Here's how the part is built. I have some questions about the finished solid (model axes, mm). Face numbers are marked on the shaded views. A direction names the side the tool comes from. Give positions to 0.01 mm unless a question says otherwise; leave off trailing zeros. Loops run counter-clockwise (first coordinate to the right, second up) from the corner with the lowest first, then second, coordinate; pieces in that order, holes last. Notation, with made-up numbers: M 0,45.25 L 44,45.25 A29 cw 44,65.25 Z; hole C 82.5,62.25 d10. An arc over 180 degrees is marked long. Answer as CSV lines item,"result". Start each with the question number.
Item 1: I want a section at C-C on z = -36.5. List the corners of the cut face in (x, y) for me (3 decimals).
Item 2: If I drill on line 1 along Y through (x, z) = (-24.25, -28) (3 decimals); line 2 along Z through (x, y) = (-21, -20); line 3 along X through (y, z) = (-4, -35), over which ranges is the centre line in solid material (lowest first)? Write a range as from..to.
Item 3: I want a section at B-B on z = -30.25. List the corners of the cut face in (x, y) for me (3 decimals), plus the area to 3 significant figures.
Item 4: For the marked faces 1, 2, 3 and 4, which set-ups out of +Z, -Z, +X, -X, +Y, -Y let a thin tool reach every point of the face, with its end or its side?
Item 5: I want a section at D-D on y = -18.75. List the corners of the cut face in (x, z) for me, plus the area to 3 significant figures.
Item 6: I want a section at A-A on y = -14.25. List the corners of the cut face in (x, z) for me.
Item 7: Will these pins go through, and if not, where does the flat tip stop? P1, Ø4, axis at x = -27, y = -10, coming from the +Z side; P2, Ø1.5, axis at y = -9, z = -29, coming from the -X side.
Item 8: If we mould it in two halves opening along Y, with no side actions, what happens to the marked faces 5, 6, 7 and 8? For each: released by +Y, released by -Y, zero draft, split by the parting line, or undercut.
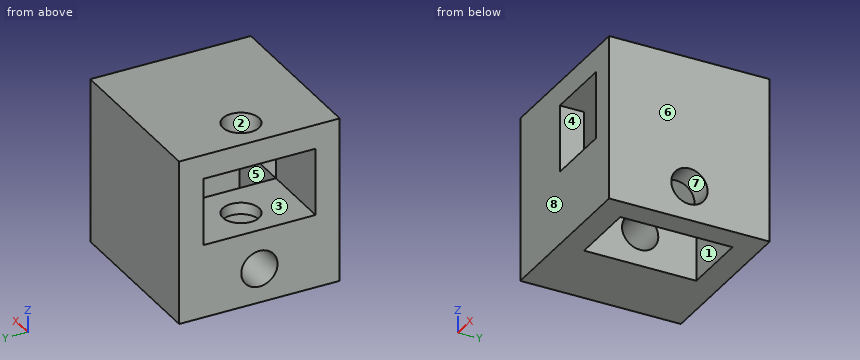
from build123d import *

# Parameters (mm, degrees)
F0_W     = 21.6662
F0_H     = 21.6662
F1_DEPTH = 3.175
F2_W     = 18.4912
F2_H     = 3.175
F2_W_2   = 9.652
F2_H_2   = 9.652
F3_DEPTH = 14.732
F5_DEPTH = 13.5382
F7_DEPTH = 25.4
F9_DEPTH = 3.175


# Not quite as in the source:
# - a length typed as a fraction of an inch, garbled in the dataset ("3 / 203.2 mm" for 3/8 in), is restored


with BuildPart() as f1:
    # F0 (on Front) → F1 (new body)
    with BuildSketch(Plane.XZ):
        with Locations((-21.4400560975, -33.0820980474)):
            Rectangle(F0_W, F0_H)
    extrude(amount=F1_DEPTH)

    # F2 (on face) → F3 (join)
    with BuildSketch(Plane.XZ.offset(3.175)):
        with Locations((-23.0275560975, -23.8364980474)):
            Rectangle(F2_W, F2_H)
        Polygon((-13.7819560975, -22.2489980474), (-13.7819560975, -25.4239980474), (-13.7819560975, -43.9151980474), (-10.6069560975, -43.9151980474), (-10.6069560975, -22.2489980474), align=None)
        with Locations((-27.4471560975, -39.0891980474)):
            Rectangle(F2_W_2, F2_H_2)
    extrude(amount=F3_DEPTH)

    # F4 (on face) → F5 (cut)
    with BuildSketch(Plane.XY.offset(-22.2489980474)):
        with BuildLine():
            ThreePointArc((-25.3961060975, -10.541), (-27.7773560975, -8.15975), (-30.1586060975, -10.541))
            ThreePointArc((-30.1586060975, -10.541), (-27.7773560975, -12.92225), (-25.3961060975, -10.541))
        make_face()
    extrude(amount=-F5_DEPTH, mode=Mode.SUBTRACT)

    # F6 (on face) → F7 (cut)
    with BuildSketch(Plane.YZ.offset(-10.6069560975)):
        with BuildLine():
            ThreePointArc((-8.15975, -39.4193980474), (-12.2247980227, -37.7356000247), (-10.541, -41.8006480474))
            ThreePointArc((-10.541, -41.8006480474), (-8.8572019773, -41.1031960701), (-8.15975, -39.4193980474))
        make_face()
    extrude(amount=-F7_DEPTH, mode=Mode.SUBTRACT)

    # F8 (on face) → F9 (join)
    with BuildSketch(Plane.XZ.offset(17.907)):
        Polygon((-10.6069560975, -43.9151980474), (-10.6069560975, -22.2489980474), (-32.2731560975, -22.2489980474), (-32.2731560975, -25.4239980474), (-22.6211560975, -25.4239980474), (-13.7819560975, -25.4239980474), (-13.7819560975, -34.2631980474), (-13.7819560975, -43.9151980474), align=None)
        Polygon((-22.6211560975, -25.4239980474), (-32.2731560975, -25.4239980474), (-32.2731560975, -43.9151980474), (-13.7819560975, -43.9151980474), (-13.7819560975, -34.2631980474), (-22.6211560975, -34.2631980474), align=None)
    extrude(amount=F9_DEPTH)


solid = f1.part
Result:
1,outline,"M -32.273,-21.082 L -10.607,-21.082 L -10.607,0 L -32.273,0 Z; hole M -22.621,-17.907 L -13.782,-17.907 L -13.782,-3.175 L -22.621,-3.175 Z"
2,line 1,"-21.082..-17.907, -3.175..0"
2,line 2,"-43.92..-34.26, -25.42..-22.25"
2,line 3,"-32.27..-22.62, -13.78..-10.61"
3,outline,"M -32.273,-21.082 L -22.621,-21.082 L -22.621,-17.907 L -32.273,-17.907 Z; M -32.273,-3.175 L -13.782,-3.175 L -13.782,-21.082 L -10.607,-21.082 L -10.607,0 L -32.273,0 Z"
3,area,"156 mm^2"
4,face 1,"none"
4,face 2,"+Z"
4,face 3,"-X"
4,face 4,"-Y"
5,outline,"M -32.27,-43.92 L -10.61,-43.92 L -10.61,-22.25 L -32.27,-22.25 Z; hole M -22.62,-34.26 L -13.78,-34.26 L -13.78,-25.42 L -22.62,-25.42 Z"
5,area,"391 mm^2"
6,outline,"M -32.27,-43.92 L -22.62,-43.92 L -22.62,-34.26 L -32.27,-34.26 Z; M -32.27,-25.42 L -13.78,-25.42 L -13.78,-43.92 L -10.61,-43.92 L -10.61,-22.25 L -32.27,-22.25 Z"
7,P1,"z = -22.25"
7,P2,"x = -13.78"
8,face 5,"undercut"
8,face 6,"zero draft"
8,face 7,"undercut"
8,face 8,"released by -Y"
